Model file for the job. Use its own axes, mm. A direction names the side the tool comes from. Round coordinates to 2 decimals unless told otherwise and drop trailing zeros. Loops run counter-clockwise (first coordinate to the right, second up) from the corner with the lowest first, then second, coordinate; pieces in that order, holes last.
from build123d import *

# Parameters (mm, degrees)
F0_R     = 12.7
F0_W     = 76.2
F0_H     = 76.2
F1_DEPTH = 25.4


with BuildPart() as f1:
    # F0 (on Right) → F1 (new body)
    with BuildSketch(Plane.YZ):
        Polygon((304.8, 0), (0, 0), (0, -203.2), (304.8, -203.2), (304.8, -76.2), align=None)
        with Locations((152.4, -177.8)):
            Circle(F0_R, mode=Mode.SUBTRACT)
        with Locations((25.4, -50.8)):
            Circle(F0_R, mode=Mode.SUBTRACT)
        with Locations((279.4, -50.8)):
            Circle(F0_R, mode=Mode.SUBTRACT)
        with Locations((342.9, -38.1)):
            Rectangle(F0_W, F0_H)
        with Locations((355.6, -50.8)):
            Circle(F0_R, mode=Mode.SUBTRACT)
    extrude(amount=F1_DEPTH)


solid = f1.part
Q1. Tool access for faces 1 (the face through (13, 381, -39)), 2 (the face through (13, 342, -76.2)): list every direction of +Z, -Z, +X, -X, +Y, -Y with a clear straight run to the whole face (end or side of a thin tool).
Q2. Probe line 1 (Y direction, x = 8, z = -40.5); line 2 (Z direction, x = 11, y = 25.4); line 3 (Y direction, x = 14.75, z = -179). List the from-to ranges inside material, lowest first.
Q3. Slice it at B-B on y = 355.6. Give the cut face in (x, z), plus the area to 3 significant figures.
Q4. Slice it at C-C on z = -50.8. Give the cut face in (x, y), plus the area to 3 significant figures.
Q5. Pull direction Z, two halves, no side cores. Call faces 3 (the face through (13, 150, -203.2)), 4 (the face through (25.4, 145, -100)), 5 (the face through (12.5, 269.3, -58.5)): pulls with the +Z half, pulls with the -Z half, needs draft (parallel to the pull), parting line crosses it, or undercut.
Q6. Flat gauge pins, fed straight in: P1, Ø20.5, axis at y = 355.6, z = -50.8, coming from the -X side; P2, Ø12.5, axis at x = 17, y = 332, coming from the -Z side; P3, Ø5, axis at x = 19, z = -86, coming from the +Y side. Where does each tip first touch, or does it go through?
Q7. Slice it at A-A on z = -177.8. Give the cut face in (x, y), plus the area to 3 significant figures.
Q8. Slice it at D-D on x = 21.5. Give the cut face in (y, z).
Reply:
1. face 1: +Z, -Z, +X, -X, +Y
1. face 2: -Z, +X, -X, +Y
2. line 1: y = 0 to 17.97, 32.83 to 271.97, 286.83 to 348.17, 363.03 to 381
2. line 2: z = -203.2 to -63.5, -38.1 to 0
2. line 3: y = 0 to 139.76, 165.04 to 304.8
3. outline: (0, -76.2) - (25.4, -76.2) - (25.4, -63.5) - (0, -63.5) - close; (0, -38.1) - (25.4, -38.1) - (25.4, 0) - (0, 0) - close
3. area: 1,290 mm2
4. outline: (0, 0) - (25.4, 0) - (25.4, 12.7) - (0, 12.7) - close; (0, 38.1) - (25.4, 38.1) - (25.4, 266.7) - (0, 266.7) - close; (0, 292.1) - (25.4, 292.1) - (25.4, 342.9) - (0, 342.9) - close; (0, 368.3) - (25.4, 368.3) - (25.4, 381) - (0, 381) - close
4. area: 7,740 mm2
5. face 3: pulls with the -Z half
5. face 4: needs draft
5. face 5: undercut
6. P1: passes through
6. P2: stops at z = -76.2
6. P3: stops at y = 304.8
7. outline: (0, 0) - (25.4, 0) - (25.4, 139.7) - (0, 139.7) - close; (0, 165.1) - (25.4, 165.1) - (25.4, 304.8) - (0, 304.8) - close
7. area: 7,100 mm2
8. outline: (0, -203.2) - (304.8, -203.2) - (304.8, -76.2) - (381, -76.2) - (381, 0) - (0, 0) - close; hole circle Ø25.4 at (25.4, -50.8); hole circle Ø25.4 at (152.4, -177.8); hole circle Ø25.4 at (279.4, -50.8); hole circle Ø25.4 at (355.6, -50.8)
